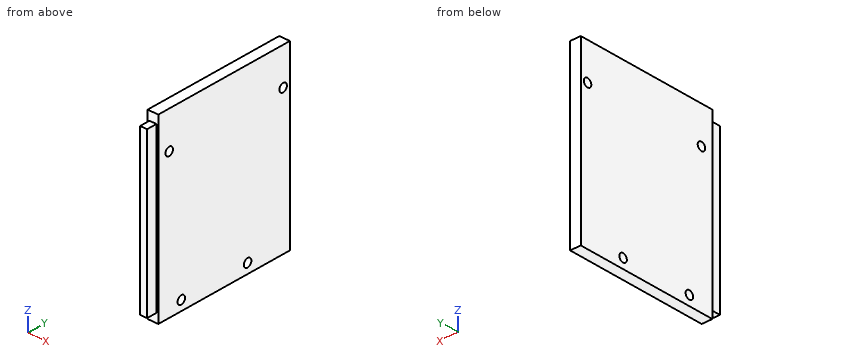
Autodesk Inventor part; units mm, degrees
ref_plane "Work Plane1" through (21.863, -4.1339, -62.2135) normal (0, 1, 0) x (-1, 0, 0)
ref_plane "YZ Plane" through (0, 0, 0) normal (1, 0, 0) x (0, 1, 0)
ref_plane "XZ Plane" through (0, 0, 0) normal (0, 1, 0) x (-1, 0, 0)
ref_plane "Work Plane1" through (21.863, -4.1339, -62.2135) normal (0, 1, 0) x (-1, 0, 0)
sketch "Sketch1" plane through (21.863, -4.1339, -62.2135) normal (0, 1, 0) x (-1, 0, 0)
  line L0 (-6.35, 34.925) -> (-6.35, -34.925) construction
  line L1 (-6.35, -34.925) -> (33.3375, -34.925) construction
  line L2 (33.3375, -34.925) -> (33.3375, 34.925) construction
  line L3 (33.3375, 34.925) -> (-6.35, 34.925) construction
  line L4 (-6.35, 34.925) -> (-6.35, -34.925)
  line L5 (-2.2016, -34.925) -> (-2.2016, 34.925)
  line L6 (-6.35, -34.925) -> (-2.2016, -34.925)
  line L7 (-6.35, 34.925) -> (-2.2016, 34.925)
  point P0 (21.863, 62.2135)
extrude "Extrusion1" add sketch "Sketch1" along normal blind 56
sketch "Sketch3" plane through (21.863, -4.1339, -62.2135) normal (0, -1, 0) x (1, 0, 0)
  line L0 (6.35, 34.925) -> (2.2016, 34.925)
  line L1 (2.2016, 34.925) -> (2.2016, -34.925)
  line L2 (2.2016, -34.925) -> (6.35, -34.925)
  line L3 (6.35, -34.925) -> (6.35, 34.925)
  line L4 (6.35, 34.925) -> (6.35, -34.925) construction
  line L5 (6.35, 0) -> (2.2016, 0) construction
  line L6 (2.2016, 34.925) -> (6.35, 34.925) construction
  line L7 (4.2758, 34.925) -> (4.2758, -34.925) construction
  line L8 (5.6258, 31.5) -> (2.9258, 31.5) construction
  line L9 (2.9258, 31.5) -> (2.9258, -31.5) construction
  line L10 (2.9258, -31.5) -> (5.6258, -31.5) construction
  line L11 (5.6258, -31.5) -> (5.6258, 31.5) construction
  line L12 (5.6258, 31.5) -> (2.9258, 31.5)
  line L13 (2.9258, 31.5) -> (2.9258, -31.5)
  line L14 (2.9258, -31.5) -> (5.6258, -31.5)
  line L15 (5.6258, -31.5) -> (5.6258, 31.5)
  line L16 (4.2758, 31.5) -> (4.2758, -31.5) construction
  line L17 (5.6258, 0) -> (2.9258, 0) construction
  point P0 (-21.863, 62.2135)
  point P1 (4.2758, 0)
  dimension "d14" = 2.7
  dimension "d15" = 63
extrude "Extrusion2" add sketch "Sketch3" along normal blind 4 contours L15 L14 L13 L12
sketch "Sketch4" plane through (28.213, -4.1339, -27.2885) normal (1, 0, 0) x (0, 0, -1)
  circle A0 centre (14.3, 53.124) radius 1.6
  circle A1 centre (14.3, 4.632) radius 1.6
  line L0 (66.1, 7.0031) -> (66.1, 9.7771) construction
  circle A2 centre (66.1, 9.7771) radius 1.6
  circle A3 centre (66.1, 38.0018) radius 1.6
  point P0 (-27.2885, 4.1339)
  dimension "d20" = 3.2
  dimension "d22" = 3.2
  dimension "d24" = 2.774
  dimension "d25" = 3.2
  dimension "d27" = 3.2
hole "Hole2" at (28.213, 48.9901, -41.5885) at (28.213, 0.4981, -41.5885) at (28.213, 5.6432, -93.3885) at (28.213, 33.8679, -93.3885) direction (-1, 0, 0) diameter 3.2 end through all
properties part number "controller_case"
Here's how the part is built. I have some questions about the finished solid (model axes, mm). Coordinates: 2 decimals unless noted, no trailing zeros. Order: outer loops, then holes, each group sorted by start corner. A loop starts at its lowest first (then second) coordinate and runs counter-clockwise, first axis right, second up.
1) Will these pins go through, and if not, where does the flat tip stop? pin 1 (2 mm diameter, centred on x = 25.5, y = -5.5, fed in from +Z); pin 2 (2 mm diameter, centred on y = -6, z = -49, fed in from -X); pin 3 (1.2 mm diameter, centred on y = -6.5, z = -72, fed in from +X).
2) Imagine slicing it at A-A on z = -76. List the corners of the cut face in (x, y) for me, and give its area (3 significant figures).
3) I need wall thicknesses on line 1 (Z direction, x = 27.7, y = 49); line 2 (Y direction, x = 25.15, z = -92.5); line 3 (Y direction, x = 27.55, z = -78). Which ranges of each line are inside material? Lowest first, please.
Response values:
1. pin 1: stops at z = -30.71
1. pin 2: stops at x = 24.79
1. pin 3: stops at x = 27.49
2. outline: (24.06, -4.13) - (24.79, -4.13) - (24.79, -8.13) - (27.49, -8.13) - (27.49, -4.13) - (28.21, -4.13) - (28.21, 51.87) - (24.06, 51.87) - close
2. area: 243 mm2
3. line 1: z = -97.14 to -43.19, -39.99 to -27.29
3. line 2: y = -8.13 to 4.31, 6.97 to 32.54, 35.2 to 51.87
3. line 3: y = -4.13 to 51.87
